from build123d import *

# Parameters (mm, degrees)
CUT_EXTRUDE1_START = 6.5
CUT_EXTRUDE1_DEPTH = 1.5


with BuildPart() as part:
    # Sketch2 → Revolve1 (revolve)
    with BuildSketch(Plane(origin=(0, 0, 0), x_dir=(0, 0, -1), z_dir=(1, 0, 0)), mode=Mode.PRIVATE) as revolve1_sk:
        with BuildLine():
            Line((6.5, 0), (6.5, 1))
            Line((6.5, 1), (6, 1.5))
            Line((6, 1.5), (-3.5, 1.5))
            Line((-3.5, 1.5), (-3.5, 2.6))
            ThreePointArc((-3.5, 2.6), (-3.543933983, 2.706066017), (-3.65, 2.75))
            Line((-3.65, 2.75), (-6.35, 2.75))
            ThreePointArc((-6.35, 2.75), (-6.456066017, 2.706066017), (-6.5, 2.6))
            Line((-6.5, 2.6), (-6.5, 0))
            Line((-6.5, 0), (6.5, 0))
        make_face()
    revolve(revolve1_sk.sketch.rotate(Axis((0, 0, -6.5), (0, 0, 1)), 90), axis=Axis((0, 0, -6.5), (0, 0, 1)))

    # Sketch3 → Cut-Extrude1 (cut)
    with BuildSketch(Plane.XY.offset(CUT_EXTRUDE1_START)):
        Polygon((-1.25, 0.721687836), (-1.25, -0.721687836), (0, -1.443375673), (1.25, -0.721687836), (1.25, 0.721687836), (0, 1.443375673), align=None)
    extrude(amount=-CUT_EXTRUDE1_DEPTH, mode=Mode.SUBTRACT)

    # Cut-Extrude2 cone 1 section (through the dimple's axis) → Cut-Extrude2 (revolve, cut)
    with BuildSketch(Plane(origin=(0, 0, 6.5), x_dir=(0, -1, 0), z_dir=(1, 0, 0))):
        Polygon((0, 0), (1.636146394, 0), (0, 0.944629561), align=None)
    revolve(axis=Axis((0, 0, 6.5), (0, 0, -1)), mode=Mode.SUBTRACT)


solid = part.part
Design review of the part built by this model. Coordinates are the model's own, in mm. A direction names the side the tool comes from. Give positions to 0.01 mm unless a question says otherwise; leave off trailing zeros. Order: outer loops, then holes, each group sorted by start corner. A loop starts at its lowest first (then second) coordinate and runs counter-clockwise, first axis right, second up.
1. For pin 1 Ø0.8 at (x, y) = (0, 0.5) entering from +Z, flat-tipped, find the tip position at first contact; note if it passes through.
Solution:
pin 1: stops at z = 5
2. To check wall thickness, follow L1, parallel to Z at x = -1.8, y = -0.9; L2, parallel to X at y = 1.15, z = 5.75; L3, parallel to Y at x = -0.45, z = 5.25. State the ranges of each line that lie inside material, in increasing order.
Solution:
L1: z = 3.5 to 6.5
L2: x = -2.5 to -0.51, 0.51 to 2.5
L3: y = -2.71 to -1.18, 1.18 to 2.71
3. Add section C-C, the plane z = -2.5. State the section outline as (x, y) points.
Solution:
outline: circle Ø3 at (0, 0)
4. Tool access review of faces 1 (the flat face through (0, 2, 3.5)), 2 (the flat face through (0, 2, 6.5)), 3 (the flat face through (-0.616, 1.088, 5.704)): name each direction out of +Z, -Z, +X, -X, +Y, -Y from which nothing blocks a thin tool from reaching the whole face with its end or side.
Solution:
face 1: -Z
face 2: +Z, +X, -X, +Y, -Y
face 3: +Z
5. Mouldability with a two-part tool opening along X and no side actions: class faces 4 (the flat face through (1.25, 0, 6)), 5 (the flat face through (0, 0, -6.5)), 6 (the cylindrical face through (-1.43, -0.45, -1.18)) as +X half, -X half, draft (parallel to the pull), parting line (faces both ways), or undercut.
Solution:
face 4: undercut
face 5: draft
face 6: parting line
6. Add section A-A, the plane z = 5.5. State the section outline as (x, y) points.
Solution:
outline: circle Ø5.5 at (0, 0); hole (-1.25, -0.72) - (0, -1.44) - (1.25, -0.72) - (1.25, 0.72) - (0, 1.44) - (-1.25, 0.72) - close
7. Add section B-B, the plane y = 0. State the section outline as (x, z) points.
Solution:
outline: (-2.75, 3.65) arc R0.15 ccw to (-2.6, 3.5) - (-1.5, 3.5) - (-1.5, -6) - (-1, -6.5) - (1, -6.5) - (1.5, -6) - (1.5, 3.5) - (2.6, 3.5) arc R0.15 ccw to (2.75, 3.65) - (2.75, 6.35) arc R0.15 ccw to (2.6, 6.5) - (1.64, 6.5) - (1.25, 6.28) - (1.25, 5) - (-1.25, 5) - (-1.25, 6.28) - (-1.64, 6.5) - (-2.6, 6.5) arc R0.15 ccw to (-2.75, 6.35) - close
